Could you check a few things on this model? Use its own coordinates, in mm. A direction names the side the tool comes from. Coordinates: 2 decimals unless noted, no trailing zeros. Order: outer loops, then holes, each group sorted by start corner. A loop starts at its lowest first (then second) coordinate and runs counter-clockwise, first axis right, second up. Notation, with made-up numbers: (57.5, 0) - (73.5, 0) arc R15 cw to (73.5, 29) - close; hole circle Ø10 at (14.25, 44.5). An arc over 180 degrees is marked (long way). Answer as a JSON object with one key per item and string values. Group by question number.
(1) Imagine slicing it at D-D, the plane y = 2.5. Give the number of separate pieces and of enclosed holes in the cut face, and give its area (3 significant figures).
(2) Imagine slicing it at C-C, the plane z = 19. Write out the boundary of the cut face in (x, y).
(3) Imagine slicing it at B-B, the plane x = 0. Write out the boundary of the cut face in (y, z).
(4) Please list where these lines run through material, in increasing order: probe 1 along Z at (x, y) = (-19, 6.75); probe 2 along X at (y, z) = (7.75, -39); probe 3 along X at (y, z) = (0.45, 0).
(5) Imagine slicing it at A-A, the plane z = 6.5. Write out the boundary of the cut face in (x, y), and give its area (3 significant figures).
(6) We'd pull the mould along X, two halves only. Please class faces 1 (the flat face through (22, 4, -29.5)), 2 (the flat face through (38.2, 8, -45.5)), 3 (the flat face through (46, 3, -1)): pulls with the +X half, pulls with the -X half, needs draft (parallel to the pull), parting line crosses it, or undercut.
(7) Will these pins go through, and if not, where does the flat tip stop? P1, Ø1.1, axis at x = -7.5, z = -45.5, coming from the +Y side; P2, Ø2, axis at x = -13, z = -35.5, coming from the +Y side.
(8) Which directions (+Z, -Z, +X, -X, +Y, -Y) give clear straight access to the entire face, cutting with the end or side of a thin tool? Please do faces 4 (the flat face through (-20, 4, 45)), 5 (the flat face through (-46, 3, 1)).
Autodesk Inventor part; units mm, degrees
ref_plane "YZ Plane" through (0, 0, 0) normal (1, 0, 0) x (0, 1, 0)
ref_plane "XZ Plane" through (0, 0, 0) normal (0, 1, 0) x (-1, 0, 0)
ref_plane "XY Plane" through (0, 0, 0) normal (0, 0, 1) x (1, 0, 0)
sketch "Sketch1" plane through (0, 0, 0) normal (0, 1, 0) x (-1, 0, 0)
  line L0 (45, 45) -> (-45, 45)
  line L1 (-45, 45) -> (-45, -45)
  line L2 (-45, -45) -> (45, -45)
  line L3 (45, -45) -> (45, 45)
  line L4 (45, 45) -> (-45, -45) construction
  line L5 (-45, 45) -> (45, -45) construction
  line L6 (-46, 46) -> (46, 46)
  line L7 (46, 46) -> (46, -46)
  line L8 (46, -46) -> (-46, -46)
  line L9 (-46, -46) -> (-46, 46)
  line L10 (-46, 46) -> (46, -46) construction
  line L11 (46, 46) -> (-46, -46) construction
  point P0 (0, 0)
  dimension "d0" = 90
  dimension "d1" = 90
  dimension "d2" = 92
  dimension "d3" = 92
extrude "Extrusion1" add sketch "Sketch1" along normal blind 1 contours L3 L2 L1 L0 | L6 L7 L8 L9
sketch "Sketch2" plane through (0, 1, 0) normal (0, 1, 0) x (1, 0, 0)
  line L0 (-46, -46) -> (46, -46)
  line L1 (46, -46) -> (46, 46)
  line L2 (46, 46) -> (-46, 46)
  line L3 (-46, 46) -> (-46, -46)
  line L4 (45, 45) -> (-45, 45)
  line L5 (-45, -20.5) -> (-45, -45)
  line L6 (-45, -45) -> (-17.75, -45)
  line L7 (45, -45) -> (45, 45)
  line L8 (45, 45) -> (-45, -45) construction
  line L9 (-45, 45) -> (45, -45) construction
  line L10 (-27.75, -30.5) -> (-17.75, -30.5)
  line L11 (-17.75, -30.5) -> (-17.75, -29.5)
  line L12 (-17.75, -29.5) -> (-27.75, -29.5)
  line L13 (-27.75, -29.5) -> (-27.75, -30.5)
  line L14 (-27.75, -30.5) -> (-26.75, -30.5)
  line L15 (-26.75, -30.5) -> (-26.75, -20.5)
  line L16 (-26.75, -20.5) -> (-27.75, -20.5)
  line L17 (-27.75, -20.5) -> (-27.75, -30.5)
  line L18 (-17.75, -45) -> (-17.75, -46)
  line L19 (-46, -46) -> (46, -46)
  line L20 (-45, -20.5) -> (-46, -20.5)
  point P0 (0, 0)
  dimension "d6" = 90
  dimension "d7" = 90
  dimension "d8" = 1
  dimension "d9" = 1
  dimension "d10" = 10
  dimension "d11" = 10
  dimension "d12" = 14.5
  dimension "d13" = 17.25
sketch "Sketch3" plane through (0, 1, 0) normal (0, 1, 0) x (1, 0, 0)
  line L0 (-27.75, -30.5) -> (-17.75, -30.5)
  line L1 (-27.75, -20.5) -> (-27.75, -30.5)
  line L2 (-26.75, -30.5) -> (-26.75, -20.5)
  line L3 (-17.75, -29.5) -> (-27.75, -29.5)
  line L4 (-26.75, -20.5) -> (-27.75, -20.5)
  line L5 (-17.75, -45) -> (-17.75, -46)
  line L6 (-45, -20.5) -> (-46, -20.5)
  line L7 (-46, 46) -> (-46, -46)
  line L8 (-45, -20.5) -> (-46, -20.5)
  line L9 (-46, -20.5) -> (-46, -46)
  line L10 (-46, -46) -> (-45, -46)
  line L11 (-45, -46) -> (-45, -20.5)
  line L12 (-46, -46) -> (46, -46)
  line L13 (-46, -46) -> (-17.75, -46)
  line L14 (-17.75, -46) -> (-17.75, -45)
  line L15 (-17.75, -45) -> (-46, -45)
  line L16 (-46, -45) -> (-46, -46)
  line L17 (-27.75, -30.5) -> (-17.75, -30.5)
  line L18 (-17.75, -30.5) -> (-17.75, -29.5)
  line L19 (-17.75, -29.5) -> (-27.75, -29.5)
  line L20 (-27.75, -29.5) -> (-27.75, -30.5)
  point P0 (0, 0)
extrude "Extrusion2" add sketch "Sketch3" along normal blind 7
sketch "Sketch4" plane through (-45, 1, 20.5) normal (0, 0, -1) x (-1, 0, 0)
  line L0 (-17.25, 0) -> (-18.25, 0)
  line L1 (-17.25, 0) -> (-17.25, 7)
  line L2 (-18.25, 7) -> (-17.25, 7)
  line L3 (-18.25, 0) -> (-18.25, 7)
  line L4 (1, 0) -> (0, 0)
  line L5 (1, 0) -> (1, 7)
  line L6 (0, 7) -> (1, 7)
  line L7 (0, 0) -> (0, 7)
  line L8 (0, 0) -> (-27.25, 0)
  arc A0 (-17.25, 4.027) -> (0, 4.027) centre (-8.625, 11.25) ccw
  line L9 (-91, 0) -> (1, 0)
  line L10 (-17.25, 0) -> (-17.25, 7)
  line L11 (-8.625, 0) -> (-17.25, 0)
  line L12 (-17.25, 0) -> (-17.25, 4.027)
  line L13 (0, 0) -> (0, 7)
  line L14 (-8.625, 0) -> (0, 0)
  line L15 (0, 0) -> (0, 4.027)
  point P0 (-45, -1)
  dimension "d16" = 22.5
  dimension "d17" = 8.625
extrude "Extrusion3" add sketch "Sketch4" against normal blind 10 contours A0 L7 L8 | L1 A0 L8
sketch "Sketch5" plane through (0, 1, 0) normal (0, 1, 0) x (1, 0, 0)
  line L0 (-17.75, -46) -> (46, -46)
  line L1 (-46, -20.5) -> (-46, -46)
  point P0 (0, 0)
  point P1 (-19, -19)
  dimension "d23" = 27
  dimension "d24" = 27
hole "Hole1" at (-19, 1, 19) direction (0, -1, 0) diameter 4 end through all
pattern_circular "Circular Pattern2" count 4 over 360 about axis through (0, -10, 0) along (0, 1, 0) of "Extrusion2", "Extrusion3", "Hole1"
sketch "Sketch6" plane through (0, 1, 0) normal (0, 1, 0) x (1, 0, 0)
  circle A0 centre (0, 0) radius 21
  dimension "d35" = 42
extrude "Extrusion4" cut sketch "Sketch6" against normal blind 10
sketch "Sketch7" plane through (0, 1, 0) normal (0, 1, 0) x (1, 0, 0)
  line L0 (45, 45) -> (-45, 45)
  line L1 (-45, 45) -> (-45, -45)
  line L2 (-45, -45) -> (45, -45)
  line L3 (45, -45) -> (45, 45)
  line L4 (45, 45) -> (-45, -45) construction
  line L5 (-45, 45) -> (45, -45) construction
  line L6 (46, -46) -> (-46, -46)
  line L7 (-46, 46) -> (46, 46)
  line L8 (46, 46) -> (46, -46)
  line L9 (46, -46) -> (-46, -46)
  line L10 (-46, -46) -> (-46, 46)
  line L11 (-46, 46) -> (46, -46) construction
  line L12 (46, 46) -> (-46, -46) construction
  point P0 (0, 0)
  dimension "d38" = 90
  dimension "d39" = 90
extrude "Extrusion5" add sketch "Sketch7" along normal blind 3
properties part number "motor_mount_base2_bottom"
Result set:
{
 "1": {"separate pieces": "5", "enclosed holes": "1", "area": "681 mm^2"},
 "2": {"outline": "(-46, 0) - (-21, 0) - (-21, 1) - (-45, 1) - (-45, 4) - (-46, 4) - close; (-17, 0) - (-8.94, 0) - (-8.94, 1) - (-17, 1) - close; (8.94, 0) - (17, 0) - (17, 1) - (8.94, 1) - close; (21, 0) - (46, 0) - (46, 8) - (45, 8) - (45, 1) - (30.5, 1) - (30.5, 8) - (29.5, 8) - (29.5, 1) - (21, 1) - close"},
 "3": {"outline": "(0, -46) - (4, -46) - (4, -45) - (1, -45) - (1, -21) - (0, -21) - close; (0, 21) - (1, 21) - (1, 45) - (4, 45) - (4, 46) - (0, 46) - close"},
 "4": {"probe 1": "z = 29.5 to 30.5, 45 to 46", "probe 2": "x = -46 to -45, 45 to 46", "probe 3": "x = -46 to -21, 21 to 46"},
 "5": {"outline": "(-46, 0) - (-19.97, 0) - (-19.97, 1) - (-45, 1) - (-45, 4) - (-46, 4) - close; (19.97, 0) - (46, 0) - (46, 4) - (45, 4) - (45, 1) - (19.97, 1) - close", "area": "58.1 mm^2"},
 "6": {"face 1": "undercut", "face 2": "needs draft", "face 3": "pulls with the +X half"},
 "7": {"P1": "stops at y = 4", "P2": "stops at y = 1"},
 "8": {"face 4": "+Y", "face 5": "+Z, -Z, -X, +Y, -Y"}
}
